For this review, take the finished solid that the model builds, in its own axes (mm). Round coordinates to 2 decimals unless told otherwise and drop trailing zeros. Order: outer loops, then holes, each group sorted by start corner. A loop starts at its lowest first (then second) coordinate and runs counter-clockwise, first axis right, second up. Notation, with made-up numbers: (-27.5, 12) -> (-10.5, 12) arc R20 cw to (-10.5, 24) -> close; hole circle Ø8 at (55.25, 12). An arc over 180 degrees is marked (long way). Answer in a Markdown table with one row per item.
```python
from build123d import *

# Parameters (mm, degrees)
F0_R     = 30.5
F0_R_2   = 27.5
F1_DEPTH = 27
F2_DEPTH = 3
F3_R     = 1.49999
F4_R     = 2.99999


# Not quite as in the source:
# - a fillet or chamfer is up to 0.001 mm smaller than in the source, because OpenCascade refuses the exact size


with BuildPart() as f1:
    # F0 (on Top) → F1 (new body)
    with BuildSketch(Plane.XY):
        Circle(F0_R)
        Circle(F0_R_2, mode=Mode.SUBTRACT)
    extrude(amount=F1_DEPTH)

    # F0 (on Top) → F2 (join)
    with BuildSketch(Plane.XY):
        Circle(F0_R)
        Circle(F0_R_2, mode=Mode.SUBTRACT)
        Circle(F0_R_2)
    extrude(amount=-F2_DEPTH)

    # F3 (radius 1.5 in the source; OpenCascade refuses exactly that, so slightly less here)
    f3_edges = [f1.edges().sort_by_distance(p)[0] for p in [
        (-30.5, 0, 27),
        (-27.5, 0, 27),
        (-27.5, 0, 0),
    ]]
    fillet(f3_edges, radius=F3_R)

    # F4 (radius 3 in the source; OpenCascade refuses exactly that, so slightly less here)
    f4_edges = [f1.edges().sort_by_distance(p)[0] for p in [
        (-30.5, 0, -3),
    ]]
    fillet(f4_edges, radius=F4_R)


solid = f1.part
```
Q1. To check wall thickness, follow probe 1 along Y at (x, z) = (0, 14); probe 2 along Z at (x, y) = (-14.5, -12). State the ranges of each line that lie inside material, in increasing order.
Answer key:
| item | result |
|---|---|
| probe 1 | y = -30.5 to -27.5, 27.5 to 30.5 |
| probe 2 | z = -3 to 0 |
Q2. The part is to be moulded in two halves that separate along Z. For faces 1 (the face through (-5.961, -26.846, 13.332)), 2 (the face through (0, 0, -3)), 3 (the face through (0, 0, 0)), say which applies: +Z half, -Z half, draft (parallel to the pull), parting line (faces both ways), or undercut.
Answer key:
| item | result |
|---|---|
| face 1 | draft |
| face 2 | -Z half |
| face 3 | +Z half |
Q3. Take a section at B-B, the plane z = 9. Write out the cut boundary in (x, y), then the cut area to 3 significant figures.
Answer key:
| item | result |
|---|---|
| outline | circle Ø61 at (0, 0); hole circle Ø55 at (0, 0) |
| area | 547 mm^2 |
Q4. Clearance check with flat-ended pins moving along their axes: pin 1 Ø6 at (y, z) = (17.5, 23.5) entering from -X; pin 2 Ø4 at (y, z) = (7.5, 18.5) entering from +X; pin 3 Ø5 at (x, z) = (-5, 23.5) entering from -Y. State where each tip first meets the part, or that it passes through.
Answer key:
| item | result |
|---|---|
| pin 1 | stops at x = -26.83 |
| pin 2 | stops at x = 30 |
| pin 3 | stops at y = -30.4 |
